```python
from build123d import *

# Parameters (mm, degrees)
F0_R     = 75
F1_DEPTH = 85
F2_SIZE2 = 25
F2_SIZE  = 20
F3_T     = -2
F4_W     = 5
F4_H     = 5
F5_DEPTH = 85.001


# Not quite as in the source:
# - the program builds the solid bodies; features that only make, move or delete a surface that nothing else refers to are left out


with BuildPart() as f1:
    # F0 (on Top) → F1 (new body)
    with BuildSketch(Plane.XY):
        Circle(F0_R)
    extrude(amount=F1_DEPTH)

    # F2
    f2_edges = [f1.edges().sort_by_distance(p)[0] for p in [
        (-75, 0, 85),
    ]]
    f2_side = f1.faces().sort_by_distance((0, 0, 85))[0]
    chamfer(f2_edges, length=F2_SIZE, length2=F2_SIZE2, reference=f2_side)

    # F3
    f3_openings = [f1.faces().sort_by_distance(p)[0] for p in [
        (0, 0, 0),
    ]]
    offset(amount=F3_T, openings=f3_openings)

    # F4 (on face) → F5 (cut, through all)
    with BuildSketch(Plane.XY.offset(85)):
        with Locations((-2.5, -2.5)):
            Rectangle(F4_W, F4_H)
    extrude(amount=-F5_DEPTH, mode=Mode.SUBTRACT)


solid = f1.part
```
Design review of the part built by this model. Coordinates are the model's own, in mm. A direction names the side the tool comes from. Give positions to 0.01 mm unless a question says otherwise; leave off trailing zeros. Loops run counter-clockwise (first coordinate to the right, second up) from the corner with the lowest first, then second, coordinate; pieces in that order, holes last. Notation, with made-up numbers: (28, -7) -> (49, -7) arc R25 cw to (49, 22) -> close; hole circle Ø4 at (-11.75, 39). An arc over 180 degrees is marked (long way). One line per item, written item: value.
Q1. We need section B-B on z = 63.5. Give the boundary of the cut face in (x, y).
Numbers:
outline: circle Ø144.4 at (0, 0); hole circle Ø139.28 at (0, 0)
Q2. For L1, parallel to Y at x = 0, z = 43; L2, parallel to Z at x = 42, y = -17; L3, parallel to Y at x = 44, z = 44, list the stretches that pass through material, from the lowest coordinate up.
Numbers:
L1: y = -75 to -73, 73 to 75
L2: z = 83 to 85
L3: y = -60.74 to -58.25, 58.25 to 60.74
Q3. We need section A-A on z = 53. Give the boundary of the cut face in (x, y), and give its area (3 significant figures).
Numbers:
outline: circle Ø150 at (0, 0); hole circle Ø146 at (0, 0)
area: 930 mm^2
Q4. For pin 1 Ø1.5 at (x, y) = (39.5, -40.5) entering from -Z; pin 2 Ø8 at (x, y) = (17, 44.5) entering from -Z; pin 3 Ø2 at (x, z) = (-3, 84.5) entering from -Y, all flat-tipped, find the tip position at first contact; note any pin that passes through.
Numbers:
pin 1: stops at z = 78.89
pin 2: stops at z = 83
pin 3: stops at y = -56.12
Q5. Draft analysis for pull direction X (two halves, no side actions). For faces 1 (the flat face through (-1, 1, 85)), 2 (the flat face through (-1, 1, 83)), 3 (the cylindrical face through (-9.764, 74.362, 29.58)), state which applies: pulls with the +X half, pulls with the -X half, needs draft (parallel to the pull), parting line crosses it, or undercut.
Numbers:
face 1: needs draft
face 2: undercut
face 3: parting line crosses it
Q6. Machinability: for faces 4 (the cylindrical face through (-15.825, -71.264, 29.234)), 5 (the flat face through (16, -72, 0)), which of the approach directions +Z, -Z, +X, -X, +Y, -Y give a long, thin tool a straight path to every point of the face, cutting with its end or side? Answer none if there is none.
Numbers:
face 4: -Z
face 5: -Z, +X, -X, +Y, -Y
